```python
from build123d import *

# Parameters (mm, degrees)
F0_R        = 21.1613086429
F1_DEPTH    = 11.9615718722
F3_DEPTH    = 11.6841569543
F4_T1_DEPTH = 36.288056526
F6_DEPTH    = 0.0834609382
F10_D       = 31.75


# Not quite as in the source:
# - a fillet or chamfer that OpenCascade refuses, or shapes differently, is made with other operations: its cross-section is extruded or revolved along the edge and cut away or added
# - the program builds the solid bodies; features that only make, move or delete a surface that nothing else refers to are left out


with BuildPart() as f1:
    # F0 (on Top) → F1 (new body)
    with BuildSketch(Plane.XY):
        Circle(F0_R)
    extrude(amount=F1_DEPTH)

    # F2 (on Top) → F3 (join)
    with BuildSketch(Plane.XY):
        Polygon((-19.0119333565, -13.1104551256), (-19.0119333565, 7.5374748558), (-36.1838054091, 6.8717853914), (-59.2216673993, 5.9786933651), (-81.0971707106, 5.1306616515), (-81.0971707106, -2.7903839946), (-62.0231479406, -13.1104551256), align=None)
    extrude(amount=F3_DEPTH)

    # F4: fillet of radius 5.08 on 1 edges, made by hand

    # F4_s2 → F4_t1 (cut)
    with BuildSketch(Plane.XY.offset(-12.3019497859)):
        with BuildLine():
            ThreePointArc((-19.0119333565, -9.2923287462), (-20.8185454842, -12.0439771445), (-23.9327132709, -13.1104551256))
            Line((-23.9327132709, -13.1104551256), (-19.0119333565, -13.1104551256))
            Line((-19.0119333565, -13.1104551256), (-19.0119333565, -9.2923287462))
        make_face()
    extrude(amount=F4_T1_DEPTH, mode=Mode.SUBTRACT)

    # F5 (on face) → F6 (join)
    with BuildSketch(Plane.XY.offset(11.6841569543)):
        with BuildLine():
            ThreePointArc((-19.0119333565, -9.2923287462), (-21.1389513114, -0.9724818434), (-19.7847977051, 7.5075137862))
            Line((-19.7847977051, 7.5075137862), (-81.0971707106, 5.1306616515))
            Line((-81.0971707106, 5.1306616515), (-81.0971707106, -2.7903839946))
            Line((-81.0971707106, -2.7903839946), (-62.0231479406, -13.1104551256))
            Line((-62.0231479406, -13.1104551256), (-23.9327132709, -13.1104551256))
            ThreePointArc((-23.9327132709, -13.1104551256), (-20.8185454842, -12.0439771445), (-19.0119333565, -9.2923287462))
        make_face()
    extrude(amount=F6_DEPTH)

    # F10 (through all)
    with Locations(Plane.XY.offset(11.9615718722)):
        with Locations((0, 0)):
            Hole(F10_D / 2)


solid = f1.part
```
Source: CAD feature listing. Evaluate the final solid. Frame: model axes, mm. A direction names the side the tool comes from. Give positions to 0.01 mm unless a question says otherwise; leave off trailing zeros. Loops run counter-clockwise (first coordinate to the right, second up) from the corner with the lowest first, then second, coordinate; pieces in that order, holes last. Notation, with made-up numbers: (79, 70) - (124, 70) arc R28 ccw to (124, 102) - close; hole circle Ø7 at (28.5, 12.5). An arc over 180 degrees is marked (long way). Use CSV: the item, a comma, the result in double quotes.
1) Cut plane A-A (y = 0). Output: boundary loops of the cut face in (x, z) (3 decimals).
Worked out:
outline,"(-81.097, 0) - (-15.875, 0) - (-15.875, 11.962) - (-21.161, 11.962) - (-21.161, 11.768) - (-81.097, 11.768) - close; (15.875, 0) - (21.161, 0) - (21.161, 11.962) - (15.875, 11.962) - close"
2) Line query: line 1 (Y direction, x = 0, z = 4.25) (3 decimals); line 2 (X direction, y = -3, z = 8.75); line 3 (X direction, y = -9, z = 10.5). Output: solid intervals per line, ascending.
Worked out:
line 1,"y = -21.161 to -15.875, 15.875 to 21.161"
line 2,"x = -80.71 to -15.59, 15.59 to 20.95"
line 3,"x = -69.62 to -13.08, 13.08 to 19.15"
3) Set-up query: faces 1 (the flat face through (-43, -13.11, 6)), 2 (the flat face through (-81.097, 1, 6)). Return all of +Z, -Z, +X, -X, +Y, -Y with unobstructed straight access to the full face (end or side cutting, diameter ignored); none if empty.
Worked out:
face 1,"+Z, -Z, -X, -Y"
face 2,"+Z, -Z, -X, +Y, -Y"
4) Cut plane C-C (z = 10). Output: boundary loops of the cut face in (x, y) (3 decimals).
Worked out:
outline,"(-81.097, -2.79) - (-62.023, -13.11) - (-23.933, -13.11) arc R5.08 ccw to (-19.012, -9.292) arc R21.161 ccw (long way) to (-19.785, 7.508) - (-81.097, 5.131) - close; hole circle Ø31.75 at (0, 0)"
5) Mould query, pull axis X, two halves, no side actions, for faces 3 (the flat face through (-31, 0, 0)), 4 (the flat face through (-71.69, -7.88, 5.8)), 5 (the cylindrical face through (3.441, -15.497, 5.897)). Classes: +X half, -X half, draft (parallel to the pull), parting line (faces both ways), or undercut.
Worked out:
face 3,"draft"
face 4,"-X half"
face 5,"undercut"
6) Cut plane B-B (x = 0). Output: boundary loops of the cut face in (y, z) (3 decimals).
Worked out:
outline,"(-21.161, 0) - (-15.875, 0) - (-15.875, 11.962) - (-21.161, 11.962) - close; (15.875, 0) - (21.161, 0) - (21.161, 11.962) - (15.875, 11.962) - close"
7) Cut plane D-D (x = 12). Output: boundary loops of the cut face in (y, z).
Worked out:
outline,"(-17.43, 0) - (-10.39, 0) - (-10.39, 11.96) - (-17.43, 11.96) - close; (10.39, 0) - (17.43, 0) - (17.43, 11.96) - (10.39, 11.96) - close"
8) Pin query (flat end, axial travel): P1, Ø1, axis at x = -2.5, z = 2, coming from the +Y side; P2, Ø16.5, axis at x = -59, y = -5, coming from the +Z side; P3, Ø3, axis at y = 14, z = 10.5, coming from the +X side; P4, Ø10, axis at x = -2.5, y = -5.5, coming from the +Z side. Return the tip coordinate at first contact, or that it passes through.
Worked out:
P1,"stops at y = 21.07"
P2,"stops at z = 11.77"
P3,"stops at x = 17.07"
P4,"passes through"
